```python
from build123d import *

# Parameters (mm, degrees)
BOSS_EXTRUDE1_DEPTH = 50.8
SKETCH2_R           = 2.5527
CUT_EXTRUDE1_DEPTH  = 50.8
SKETCH3_R           = 2.5527
CUT_EXTRUDE2_DEPTH  = 50.8
SKETCH4_R           = 9.525
CUT_EXTRUDE3_DEPTH  = 3.175


with BuildPart() as part:
    # Sketch1 → Boss-Extrude1 (new body)
    with BuildSketch(Plane.XY):
        Polygon((0, 0), (-3.175, 0), (-3.175, 53.975), (0, 53.975), (0, 3.175), (73.025, 3.175), (73.025, 0), align=None)
    extrude(amount=BOSS_EXTRUDE1_DEPTH)

    # Sketch2 → Cut-Extrude1 (cut)
    with BuildSketch(Plane(origin=(0, 0, 0), x_dir=(0, 0, -1), z_dir=(1, 0, 0))):
        with Locations((-25.4, 41.275)):
            Circle(SKETCH2_R)
        with Locations((-38.1, 15.875)):
            Circle(SKETCH2_R)
        with Locations((-12.7, 15.875)):
            Circle(SKETCH2_R)
    extrude(amount=-CUT_EXTRUDE1_DEPTH, mode=Mode.SUBTRACT)

    # Sketch3 → Cut-Extrude2 (cut)
    with BuildSketch(Plane(origin=(0, 3.175, 0), x_dir=(1, 0, 0), z_dir=(0, 1, 0))):
        with Locations((60.325, -25.4)):
            Circle(SKETCH3_R)
        with Locations((34.925, -12.7)):
            Circle(SKETCH3_R)
        with Locations((34.925, -38.1)):
            Circle(SKETCH3_R)
    extrude(amount=-CUT_EXTRUDE2_DEPTH, mode=Mode.SUBTRACT)

    # Sketch4 → Cut-Extrude3 (cut)
    with BuildSketch(Plane(origin=(0, 0, 0), x_dir=(0, 0, -1), z_dir=(1, 0, 0))):
        with Locations((-25.4, 25.4)):
            Circle(SKETCH4_R)
    extrude(amount=-CUT_EXTRUDE3_DEPTH, mode=Mode.SUBTRACT)


solid = part.part
```
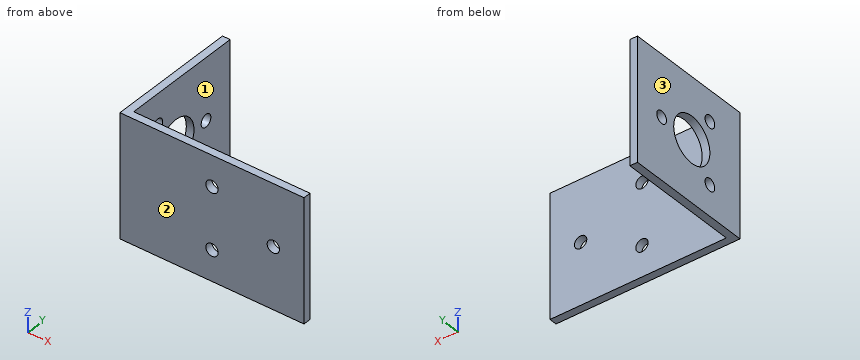
The listing builds one solid part. Answer for the finished solid, in the listing's coordinates (mm). Face numbers are marked on the shaded views. Round coordinates to 2 decimals unless told otherwise and drop trailing zeros. Order: outer loops, then holes, each group sorted by start corner. A loop starts at its lowest first (then second) coordinate and runs counter-clockwise, first axis right, second up. Notation, with made-up numbers: (21, 77.5) - (48, 77.5) arc R15 ccw to (48, 89.5) - close; hole circle Ø4 at (-24, 50.5). An arc over 180 degrees is marked (long way). Put each result on its own line as item: value. Start each with the question number.
(1) Determine the mould class of the marked faces 1, 2 and 3 for opening direction X: released by +X, released by -X, zero draft, split by the parting line, or undercut.
(2) Straight lines are drawn through the part: probe 1 along Y at (x, z) = (-1.3, 25.4) (3 decimals); probe 2 along X at (y, z) = (1.9, 38.1) (3 decimals); probe 3 along X at (y, z) = (4, 21) (3 decimals). For each, find the intervals that lie inside material, in ascending order. Write a range as from..to.
(3) Find section A-A (y = 25.4). Give the vertices of the cut face in (x, z) (3 decimals).
(4) Find section B-B (z = 38.1). Give the vertices of the cut face in (x, y) (3 decimals), plus the area to 3 significant figures.
(5) Given P1, Ø15, axis at x = 35.5, z = 28, coming from the +Y side (3 decimals); P2, Ø2, axis at y = 39.5, z = 16, coming from the +X side, each flat-ended and moving along its own axis, determine where each tip first touches the part or whether it passes through.
(6) Find section C-C (z = 25.4). Give the vertices of the cut face in (x, y) (3 decimals).
(7) Find section D-D (x = 35). Give the vertices of the cut face in (y, z) (3 decimals).
Reply:
1. face 1: released by +X
1. face 2: zero draft
1. face 3: released by -X
2. probe 1: 0..15.875, 34.925..38.722, 43.828..53.975
2. probe 2: -3.175..32.372, 37.478..73.025
2. probe 3: -3.175..0
3. outline: (-3.175, 0) - (0, 0) - (0, 15.875) - (-3.175, 15.875) - close; (-3.175, 34.925) - (0, 34.925) - (0, 50.8) - (-3.175, 50.8) - close
4. outline: (-3.175, 0) - (32.372, 0) - (32.372, 3.175) - (0, 3.175) - (0, 13.322) - (-3.175, 13.322) - close; (-3.175, 18.428) - (0, 18.428) - (0, 53.975) - (-3.175, 53.975) - close; (37.478, 0) - (73.025, 0) - (73.025, 3.175) - (37.478, 3.175) - close
4. area: 371 mm^2
5. P1: y = 3.175
5. P2: x = 0
6. outline: (-3.175, 0) - (57.772, 0) - (57.772, 3.175) - (0, 3.175) - (0, 15.875) - (-3.175, 15.875) - close; (-3.175, 34.925) - (0, 34.925) - (0, 38.722) - (-3.175, 38.722) - close; (-3.175, 43.828) - (0, 43.828) - (0, 53.975) - (-3.175, 53.975) - close; (62.878, 0) - (73.025, 0) - (73.025, 3.175) - (62.878, 3.175) - close
7. outline: (0, 0) - (3.175, 0) - (3.175, 10.148) - (0, 10.148) - close; (0, 15.252) - (3.175, 15.252) - (3.175, 35.548) - (0, 35.548) - close; (0, 40.652) - (3.175, 40.652) - (3.175, 50.8) - (0, 50.8) - close
